```python
from build123d import *

# Parameters (mm, degrees)
SKETCH1_R               = 1.25
BOSS_EXTRUDE1_DEPTH     = 5
SKETCH2_R               = 1.25
CUT_EXTRUDE1_DEPTH      = 5
CUT_EXTRUDE2_DEPTH      = 14.693063938
CUT_EXTRUDE2_DEPTH_BACK = 14.693063938
SKETCH4_W               = 5
SKETCH4_H               = 5
SKETCH5_W               = 5
SKETCH5_H               = 1.5
CUT_EXTRUDE3_DEPTH      = 1.25
SKETCH6_R               = 0.2
CUT_EXTRUDE4_DEPTH      = 12.456439237
FILLET1_R               = 0.5
SKETCH7_W               = 5
SKETCH7_H               = 10
BOSS_EXTRUDE2_DEPTH     = 10
SKETCH9_R               = 1.25
CUT_EXTRUDE6_DEPTH      = 10
SKETCH11_W              = 5
SKETCH11_H              = 20
CUT_EXTRUDE7_DEPTH      = 10
FILLET3_R               = 2.5


with BuildPart() as part:
    # Sketch1 → Boss-Extrude1 (new, symmetric)
    with BuildSketch(Plane.XY):
        with BuildLine():
            ThreePointArc((2.5, 0), (-1.767766953, 1.767766953), (0, -2.5))
            Line((0, -2.5), (10, -2.5))
            ThreePointArc((10, -2.5), (11.767766953, 1.767766953), (7.5, 0))
            Line((7.5, 0), (2.5, 0))
        make_face()
        with Locations((10, 0)):
            Circle(SKETCH1_R, mode=Mode.SUBTRACT)
        Circle(SKETCH1_R, mode=Mode.SUBTRACT)
    extrude(amount=BOSS_EXTRUDE1_DEPTH, both=True)

    # Sketch2 → Cut-Extrude1 (cut)
    with BuildSketch(Plane(origin=(0, 0, 0), x_dir=(1, 0, 0), z_dir=(0, 1, 0))):
        with Locations(Location((5, 0, 0), (0, 0, 270))):
            Circle(SKETCH2_R)
    extrude(amount=-CUT_EXTRUDE1_DEPTH, mode=Mode.SUBTRACT)

    # Sketch4 → Cut-Extrude2 (cut, two sides: drawn at the far end of the back side and taken through both)
    with BuildSketch(Plane(origin=(0, 0, 0), x_dir=(1, 0, 0), z_dir=(0, 1, 0)).offset(-CUT_EXTRUDE2_DEPTH_BACK)):
        Rectangle(SKETCH4_W, SKETCH4_H)
        with Locations((10, 0)):
            Rectangle(SKETCH4_W, SKETCH4_H)
    extrude(amount=CUT_EXTRUDE2_DEPTH + CUT_EXTRUDE2_DEPTH_BACK, mode=Mode.SUBTRACT)

    # Sketch5 → Cut-Extrude3 (cut)
    with BuildSketch(Plane(origin=(0, 0, 0), x_dir=(1, 0, 0), z_dir=(0, 1, 0))):
        with Locations((5, 0)):
            Rectangle(SKETCH5_W, SKETCH5_H)
    extrude(amount=-CUT_EXTRUDE3_DEPTH, mode=Mode.SUBTRACT)

    # Sketch6 → Cut-Extrude4 (cut, through all)
    with BuildSketch(Plane(origin=(7.5, 0, 0), x_dir=(0, 0, -1), z_dir=(1, 0, 0))):
        with Locations((0, -1.875)):
            Circle(SKETCH6_R)
        with Locations((1, -1.875)):
            Circle(SKETCH6_R)
        with Locations((2, -1.875)):
            Circle(SKETCH6_R)
        with Locations((-1, -1.875)):
            Circle(SKETCH6_R)
        with Locations((-2, -1.875)):
            Circle(SKETCH6_R)
    extrude(amount=-CUT_EXTRUDE4_DEPTH, mode=Mode.SUBTRACT)

    # Fillet1
    fillet1_edges = [part.edges().sort_by_distance(p)[0] for p in [
        (6.75, -1.25, 0.75),
        (3.25, -1.25, 0.75),
        (3.25, -1.25, -0.75),
        (6.75, -1.25, -0.75),
        (6.75, 0, 0.75),
        (6.75, 0, -0.75),
        (3.25, 0, 0.75),
        (3.25, 0, -0.75),
    ]]
    fillet(fillet1_edges, radius=FILLET1_R - 0.0001)  # a hair under: the kernel refuses the full size

    # Sketch7 → Boss-Extrude2 (add)
    with BuildSketch(Plane.XY.offset(5)):
        with Locations((5, -7.5)):
            Rectangle(SKETCH7_W, SKETCH7_H)
    extrude(amount=-BOSS_EXTRUDE2_DEPTH)

    # Sketch9 → Cut-Extrude6 (cut)
    with BuildSketch(Plane(origin=(0, 0, -5), x_dir=(-1, 0, 0), z_dir=(0, 0, -1))):
        with Locations((-5, -7.5)):
            Circle(SKETCH9_R)
    extrude(amount=-CUT_EXTRUDE6_DEPTH, mode=Mode.SUBTRACT)

    # Sketch11 → Cut-Extrude7 (cut)
    with BuildSketch(Plane(origin=(7.5, 0, 0), x_dir=(0, 0, -1), z_dir=(1, 0, 0))):
        with Locations((0, -12.5)):
            Rectangle(SKETCH11_W, SKETCH11_H)
    extrude(amount=-CUT_EXTRUDE7_DEPTH, mode=Mode.SUBTRACT)

    # Fillet3
    fillet3_edges = [part.edges().sort_by_distance(p)[0] for p in [
        (2.5, -12.5, 3.75),
        (7.5, -12.5, 3.75),
        (2.5, -12.5, -3.75),
        (7.5, -12.5, -3.75),
    ]]
    fillet(fillet3_edges, radius=FILLET3_R - 0.0001)  # a hair under: the kernel refuses the full size


solid = part.part
```
For this review, take the finished solid that the model builds, in its own axes (mm). A direction names the side the tool comes from. Coordinates: 2 decimals unless noted, no trailing zeros. Write each loop counter-clockwise with the first axis right and the second up, starting at its lowest first coordinate (ties: lowest second). Pieces come first, ordered by that corner, then holes.
(1) Tool access review of faces 4 (the face through (1, -1, 2.5)), 5 (the face through (4, -6, -2.5)), 6 (the face through (7.5, -6, 4)), 7 (the face through (5, 0, 3)): name each direction out of +Z, -Z, +X, -X, +Y, -Y from which nothing blocks a thin tool from reaching the whole face with its end or side.
(2) Add section B-B on y = -6.75. Give the boundary of the cut face in (x, z), then the cut area to 3 significant figures.
(3) The part is to be moulded in two halves that separate along Y. For faces 1 (the face through (5, -3, 5)), 2 (the face through (-1.709, 1.825, -3.732)), 3 (the face through (5.27, -8.72, -3.77)), say which applies: +Y half, -Y half, draft (parallel to the pull), parting line (faces both ways), or undercut.
(4) For pin 1 Ø1.3 at (y, z) = (-1.5, 0) entering from +X; pin 2 Ø2.5 at (x, y) = (10.5, -0.5) entering from -Z; pin 3 Ø3 at (x, z) = (5, 0) entering from +Y; pin 4 Ø1.5 at (x, y) = (0, 0) entering from -Z, all flat-tipped, find the tip position at first contact; note any pin that passes through.
(5) Add section D-D on z = 4.25. Count the separate pieces of the cut face and the enclosed holes in it, then the cut area to 3 significant figures.
(6) Add section C-C on z = 2. Give the boundary of the cut face in (x, y) (3 decimals).
(7) Add section A-A on z = 0. Give the boundary of the cut face in (x, y) (3 decimals), then the cut area to 4 significant figures.
(8) Wall thickness on probe 1 along X at (y, z) = (0.5, -3.5); probe 2 along X at (y, z) = (-7.75, 2.75); probe 3 along Z at (x, y) = (11.25, -1): over which ranges is each line inside the solid? List them lowest first.
Answer sheet:
1. face 4: -X, +Y, -Y
1. face 5: +X, -X, -Y
1. face 6: +Z, -Z, +X, -Y
1. face 7: +Z, -Z, +Y
2. outline: (2.5, -5) - (4, -5) - (4, -2.5) - (2.5, -2.5) - close; (2.5, 2.5) - (4, 2.5) - (4, 5) - (2.5, 5) - close; (6, -5) - (7.5, -5) - (7.5, -2.5) - (6, -2.5) - close; (6, 2.5) - (7.5, 2.5) - (7.5, 5) - (6, 5) - close
2. area: 15.0 mm2
3. face 1: draft
3. face 2: parting line
3. face 3: undercut
4. pin 1: stops at x = 7.5
4. pin 2: stops at z = -5
4. pin 3: stops at y = 0
4. pin 4: passes through
5. separate pieces: 1
5. enclosed holes: 3
5. area: 87.0 mm2
6. outline: (2.5, -2.5) - (7.5, -2.5) - (7.5, -2.075) - (2.5, -2.075) - close; (2.5, -1.675) - (7.5, -1.675) - (7.5, 0) - (2.5, 0) - close
7. outline: (2.5, -2.5) - (3.75, -2.5) - (3.75, -2.075) - (2.5, -2.075) - close; (2.5, -1.675) - (3.75, -1.675) - (3.75, -1.25) - (2.5, -1.25) - close; (6.25, -2.5) - (7.5, -2.5) - (7.5, -2.075) - (6.25, -2.075) - close; (6.25, -1.675) - (7.5, -1.675) - (7.5, -1.25) - (6.25, -1.25) - close
7. area: 2.125 mm2
8. probe 1: x = -2.45 to -1.15, 1.15 to 2.45, 7.55 to 8.85, 11.15 to 12.45
8. probe 2: x = 2.5 to 3.78, 6.22 to 7.5
8. probe 3: z = -5 to -2.5, 2.5 to 5
